from build123d import *

# Parameters (mm, degrees)
SKETCH1_W               = 69
SKETCH1_H               = 14
BOSS_EXTRUDE1_DEPTH     = 2
SKETCH2_W               = 52.910547302
SKETCH2_H               = 2
BOSS_EXTRUDE2_DEPTH     = 4
CUT_EXTRUDE1_DEPTH      = 20
CUT_EXTRUDE1_DEPTH_BACK = 20
CUT_EXTRUDE2_DEPTH      = 2
BOSS_EXTRUDE3_DEPTH     = 2
BOSS_EXTRUDE4_DEPTH     = 4
BOSS_EXTRUDE5_DEPTH     = 6
CUT_EXTRUDE3_DEPTH      = 6
BOSS_EXTRUDE6_START     = -16.09
BOSS_EXTRUDE6_DEPTH     = 2
CUT_EXTRUDE4_DEPTH      = 20
CUT_EXTRUDE4_DEPTH_BACK = 20
SKETCH11_W              = 60.759047224
SKETCH11_H              = 31.87532725


with BuildPart() as part:
    # Sketch1 → Boss-Extrude1 (new body)
    with BuildSketch(Plane.XY):
        with Locations((-11.678861789, -0.654471545)):
            Rectangle(SKETCH1_W, SKETCH1_H)
    extrude(amount=BOSS_EXTRUDE1_DEPTH)

    # Sketch2 → Boss-Extrude2 (add)
    with BuildSketch(Plane.XY.offset(2)):
        with Locations((-19.723588138, 5.345528455)):
            Rectangle(SKETCH2_W, SKETCH2_H)
    extrude(amount=BOSS_EXTRUDE2_DEPTH)

    # Sketch4 → Cut-Extrude1 (cut, two sides: drawn at the far end of the back side and taken through both)
    with BuildSketch(Plane(origin=(0, 6.345528455, 0), x_dir=(1, 0, 0), z_dir=(0, 1, 0)).offset(-CUT_EXTRUDE1_DEPTH_BACK)):
        Polygon((-18.178861789, 0), (-33.809396177, -6), (-46.178861789, -6), (-46.178861789, 0), align=None)
    extrude(amount=CUT_EXTRUDE1_DEPTH + CUT_EXTRUDE1_DEPTH_BACK, mode=Mode.SUBTRACT)

    # Sketch5 → Cut-Extrude2 (cut)
    with BuildSketch(Plane(origin=(0, 6.345528455, 0), x_dir=(1, 0, 0), z_dir=(0, 1, 0))):
        Polygon((-33.809396177, -6), (-23.38959077, -2.000211452), (-21.854215798, -6), align=None)
    extrude(amount=-CUT_EXTRUDE2_DEPTH, mode=Mode.SUBTRACT)

    # Sketch6 → Boss-Extrude3 (add)
    with BuildSketch(Plane.XY.offset(2)):
        Polygon((6.731685513, 6.345528455), (22.821685513, 22.435528455), (22.821138211, 6.345528455), align=None)
    extrude(amount=-BOSS_EXTRUDE3_DEPTH)

    # Sketch7 → Boss-Extrude4 (add)
    with BuildSketch(Plane.XY.offset(2)):
        Polygon((6.731685513, 4.345528455), (22.821617483, 20.435528456), (22.821685513, 22.435528455), (6.731685513, 6.345528455), align=None)
    extrude(amount=BOSS_EXTRUDE4_DEPTH)

    # Sketch8 → Boss-Extrude5 (add)
    with BuildSketch(Plane.XY.offset(6)):
        Polygon((22.821685513, 22.435528455), (6.731685513, 6.345528455), (-21.854215798, 6.345528455), (-21.854215798, 4.345528455), (6.731685513, 4.345528455), (22.821617483, 20.435528456), align=None)
    extrude(amount=BOSS_EXTRUDE5_DEPTH)

    # Sketch9 → Cut-Extrude3 (cut)
    with BuildSketch(Plane.XZ.offset(-4.345528455)):
        Polygon((-23.389039918, 2), (-21.854215798, 6), (-19.551979619, 12), (-21.854215798, 12), align=None)
    extrude(amount=-CUT_EXTRUDE3_DEPTH, mode=Mode.SUBTRACT)


with BuildPart() as cut_extrude3_piece_1:
    # of the separate pieces the step leaves, piece 1, a body of its own (cut_extrude3_pieces)
    add(part.part.solids().sort_by_distance((-18.178861789, 6.345528455, 0))[0])

    # Sketch10 → Boss-Extrude6 (add)
    with BuildSketch(Plane.XZ.offset(-4.345528455).offset(BOSS_EXTRUDE6_START)):
        Polygon((22.821617483, 12), (24.765438688, 12), (22.821138211, 2), align=None)
    extrude(amount=-BOSS_EXTRUDE6_DEPTH)


with BuildPart() as cut_extrude3_piece_2:
    # of the separate pieces the step leaves, piece 2, a body of its own (cut_extrude3_pieces)
    add(part.part.solids().sort_by_distance((-23.38861886, 6.345528455, 2.002743364))[0])


with BuildPart() as body_3:
    # Mirror1: mirrored copy
    add(cut_extrude3_piece_1.part.mirror(Plane(origin=(-46.178861789, -7.654471545, 2), x_dir=(0, 0, 1), z_dir=(0, 1, 0))))


with BuildPart() as cut_extrude4_tool:
    # Sketch11 → Cut-Extrude4 (new, two sides: drawn at the far end of the back side and taken through both)
    with BuildSketch(Plane.XY.offset(2).offset(-CUT_EXTRUDE4_DEPTH_BACK)):
        with Locations((3.114590222, 8.28319208)):
            Rectangle(SKETCH11_W, SKETCH11_H)
    extrude(amount=CUT_EXTRUDE4_DEPTH + CUT_EXTRUDE4_DEPTH_BACK)


with BuildPart() as cut_extrude3_piece_1_1:
    add(cut_extrude3_piece_1.part)

    # Cut-Extrude4: cut by cut_extrude4_tool
    add(cut_extrude4_tool.part, mode=Mode.SUBTRACT)


with BuildPart() as cut_extrude3_piece_2_1:
    add(cut_extrude3_piece_2.part)

    # Cut-Extrude4: cut by cut_extrude4_tool
    add(cut_extrude4_tool.part, mode=Mode.SUBTRACT)


solid = body_3.part
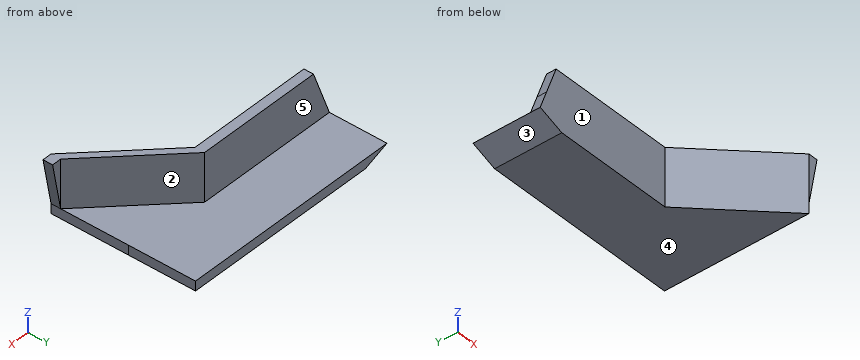
Read the model definition and answer for the solid it produces. Units are mm, in the model's axes. Face numbers are marked on the shaded views. A direction names the side the tool comes from. Coordinates: 2 decimals unless noted, no trailing zeros. Loops run counter-clockwise (first coordinate to the right, second up) from the corner with the lowest first, then second, coordinate; pieces in that order, holes last.
Q1. The part is cut by section C-C on y = -28.5. Write down the section's boundary in (x, z).
Q2. Which of the six approach directions +Z, -Z, +X, -X, +Y, -Y give full straight-line access (tool end or side, diameter ignored) to the marked faces 1, 2, 3, 4 and 5?
Q3. Consider probe 1 along Z at (x, y) = (16.5, -16); probe 2 along Y at (x, z) = (-18, 10.75); probe 3 along Y at (x, z) = (0.5, 1.75). Determine where each line is inside the solid, lowest interval first.
Q4. Each of these flat-tipped pins is pushed along its axis until it touches: pin 1 Ø5 at (x, y) = (-15.5, -15.5) entering from +Z; pin 2 Ø0.6 at (y, z) = (-17, 1) entering from +X; pin 3 Ø4 at (x, z) = (-7.5, 11) entering from -Y; pin 4 Ø0.6 at (x, z) = (24.5, 6.5) entering from +Y. Where does it stop, or does it pass through?
Q5. The part is cut by section B-B on x = 4.5. Write down the section's boundary in (y, z), and give its area (3 significant figures).
Results below:
1. outline: (13.58, 0) - (22.82, 0) - (22.82, 2) - (15.58, 2) - (15.58, 12) - (13.58, 12) - close
2. face 1: +Z, -Z, -X, -Y
2. face 2: +Z, +X, +Y
2. face 3: -Z, -X, +Y, -Y
2. face 4: -Z, +X, -X, +Y, -Y
2. face 5: +Z, +X, -X, +Y
3. probe 1: z = 0 to 2
3. probe 2: y = -21.65 to -19.65
3. probe 3: y = -21.65 to -7.65
4. pin 1: stops at z = 2
4. pin 2: stops at x = 22.82
4. pin 3: stops at y = -21.65
4. pin 4: passes through
5. outline: (-21.65, 0) - (-7.65, 0) - (-7.65, 2) - (-19.65, 2) - (-19.65, 12) - (-21.65, 12) - close
5. area: 48.0 mm2
